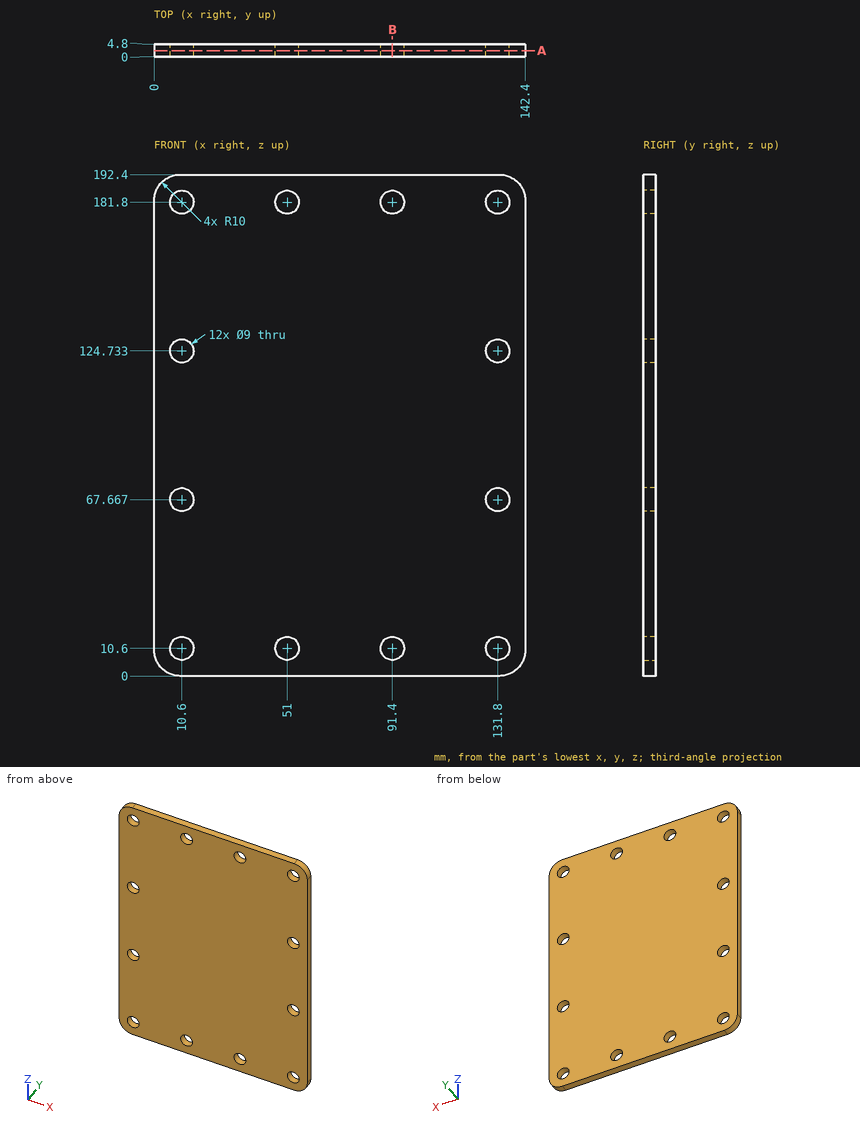
Can you work these out from the drawing? Everything is in mm from the part's minimum corner. Round coordinates to 2 decimals unless told otherwise and drop trailing zeros. Loops run counter-clockwise (first coordinate to the right, second up) from the corner with the lowest first, then second, coordinate; pieces in that order, holes last. Notation, with made-up numbers: M -14.5,74 L 42.5,74 A17 ccw 42.5,106 Z; hole C 26.5,8.25 d1. An arc over 180 degrees is marked long. Write item = value, one per line.
1. I need wall thicknesses on probe 1 along X at (y, z) = (2.4, 10.6); probe 2 along Z at (x, y) = (13, 2.95); probe 3 along X at (y, z) = (4, 128.5). Which ranges of each line are inside material? Lowest first, please.
Results below:
probe_1 = 0 to 6.1, 15.1 to 46.5, 55.5 to 86.9, 95.9 to 127.3, 136.3 to 142.4
probe_2 = 0 to 6.79, 14.41 to 63.86, 71.47 to 120.93, 128.54 to 177.99, 185.61 to 192.4
probe_3 = 0 to 8.14, 13.06 to 129.34, 134.26 to 142.4
2. I want a section at B-B, the plane x = 91.4. Write out the boundary of the cut face in (y, z), and give its area (3 significant figures).
Results below:
outline = M 0,0 L 4.8,0 L 4.8,6.1 L 0,6.1 Z; M 0,15.1 L 4.8,15.1 L 4.8,177.3 L 0,177.3 Z; M 0,186.3 L 4.8,186.3 L 4.8,192.4 L 0,192.4 Z
area = 837 mm²
3. Will this pin go through, and if not, where does the flat tip stop? P1, Ø8, axis at x = 91.4, z = 10.6, coming from the -Y side.
Results below:
P1 = through
4. I want a section at A-A, the plane y = 2.3. Count the separate pieces of the cut face and the enclosed holes in it, and give its area (3 significant figures).
Results below:
separate_pieces = 1
enclosed_holes = 12
area = 26,500 mm²
